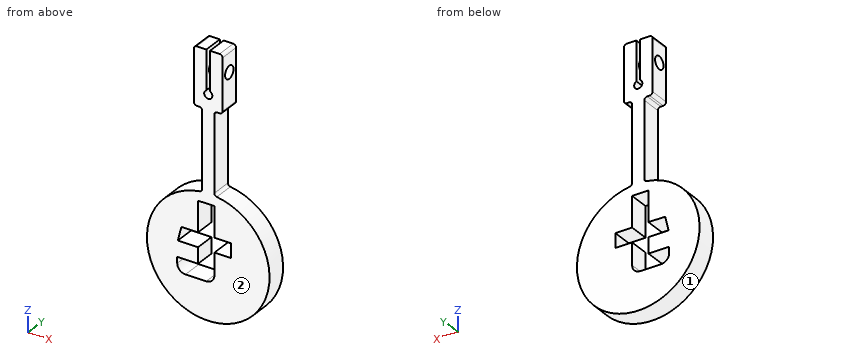
```python
from build123d import *

# Parameters (mm, degrees)
BOSS_EXTRUDE2_DEPTH = 5
SKETCH5_R           = 1.55
CUT_EXTRUDE1_DEPTH  = 60.905859109
FILLET6_R           = 0.7
FILLET7_R           = 0.7
FILLET8_R           = 0.7
FILLET9_R           = 0.7
FILLET10_R          = 0.7
FILLET11_R          = 0.7
FILLET12_R          = 0.7
FILLET13_R          = 0.7
FILLET14_R          = 2
FILLET15_R          = 2


with BuildPart() as part:
    # Sketch3 → Boss-Extrude2 (new body)
    with BuildSketch(Plane(origin=(0, 0, 0), x_dir=(1, 0, 0), z_dir=(0, 1, 0))):
        with BuildLine():
            Line((0.454624582, 2.591384664), (0.454624582, -7))
            Line((0.454624582, -7), (3.5, -7))
            Line((3.5, -7), (3.5, 7))
            Line((3.5, 7), (1.5, 7))
            Line((1.5, 7), (1.5, 26.833112609))
            ThreePointArc((1.5, 26.833112609), (0, 56.757924165), (-1.5, 26.833112609))
            Line((-1.5, 26.833112609), (-1.5, 7))
            Line((-1.5, 7), (-3.5, 7))
            Line((-3.5, 7), (-3.5, -7))
            Line((-3.5, -7), (-0.454624582, -7))
            Line((-0.454624582, -7), (-0.454624582, 2.591384664))
            ThreePointArc((-0.454624582, 2.591384664), (0, 4.482067823), (0.454624582, 2.591384664))
        make_face()
        Polygon((1.5, 36.708863036), (1.5, 29.251163785), (-2.5, 29.251163785), (-2.5, 36.708863036), (-6.573288639, 36.708863036), (-7.435532145, 40.208863036), (-2.5, 40.208863036), (-2.5, 44.101325286), (-7.582366619, 44.101325286), (-7.582366619, 47.601325286), (1.5, 47.601325286), (1.5, 40.208863036), (5.609756824, 40.208863036), (5.609756824, 36.708863036), align=None, mode=Mode.SUBTRACT)
    extrude(amount=BOSS_EXTRUDE2_DEPTH)

    # Sketch5 → Cut-Extrude1 (cut, through all)
    with BuildSketch(Plane.ZY.offset(3.5)):
        with Locations((1.710892138, 2.5)):
            Circle(SKETCH5_R)
    extrude(amount=-CUT_EXTRUDE1_DEPTH, mode=Mode.SUBTRACT)

    # Fillet6
    fillet6_edges = [part.edges().sort_by_distance(p)[0] for p in [
        (1.5, 2.5, -7),
    ]]
    fillet(fillet6_edges, radius=FILLET6_R)

    # Fillet7
    fillet7_edges = [part.edges().sort_by_distance(p)[0] for p in [
        (3.5, 2.5, -7),
    ]]
    fillet(fillet7_edges, radius=FILLET7_R)

    # Fillet8
    fillet8_edges = [part.edges().sort_by_distance(p)[0] for p in [
        (-1.5, 2.5, -7),
    ]]
    fillet(fillet8_edges, radius=FILLET8_R)

    # Fillet9
    fillet9_edges = [part.edges().sort_by_distance(p)[0] for p in [
        (-3.5, 2.5, -7),
    ]]
    fillet(fillet9_edges, radius=FILLET9_R)

    # Fillet10
    fillet10_edges = [part.edges().sort_by_distance(p)[0] for p in [
        (3.5, 2.5, 7),
    ]]
    fillet(fillet10_edges, radius=FILLET10_R)

    # Fillet11
    fillet11_edges = [part.edges().sort_by_distance(p)[0] for p in [
        (-3.5, 2.5, 7),
    ]]
    fillet(fillet11_edges, radius=FILLET11_R)

    # Fillet12
    fillet12_edges = [part.edges().sort_by_distance(p)[0] for p in [
        (1.5, 2.5, -26.833112609),
    ]]
    fillet(fillet12_edges, radius=FILLET12_R)

    # Fillet13
    fillet13_edges = [part.edges().sort_by_distance(p)[0] for p in [
        (-1.5, 2.5, -26.833112609),
    ]]
    fillet(fillet13_edges, radius=FILLET13_R)

    # Fillet14
    fillet14_edges = [part.edges().sort_by_distance(p)[0] for p in [
        (1.5, 2.5, -47.601325286),
    ]]
    fillet(fillet14_edges, radius=FILLET14_R)

    # Fillet15
    fillet15_edges = [part.edges().sort_by_distance(p)[0] for p in [
        (-7.582366619, 2.5, -47.601325286),
    ]]
    fillet(fillet15_edges, radius=FILLET15_R)


solid = part.part
```
The listing builds one solid part. Answer for the finished solid, in the listing's coordinates (mm). Face numbers are marked on the shaded views. Round coordinates to 2 decimals unless told otherwise and drop trailing zeros. Loops run counter-clockwise (first coordinate to the right, second up) from the corner with the lowest first, then second, coordinate; pieces in that order, holes last.
Q1. Section B-B, the plane x = -5 is taken. Determine the outline of the cut face in (y, z).
Q2. Section C-C, the plane y = 2.5 is taken. Count the separate pieces of the cut face and the enclosed holes in it, then the cut area to 3 significant figures.
Q3. Section D-D, the plane z = -33 is taken. Determine the outline of the cut face in (x, y).
Q4. Section A-A, the plane z = -43.5 is taken. Determine the outline of the cut face in (x, y).
Q5. For a pull along X with two mould halves and no side action, classify the marked faces 1 and 2 as released by +X, released by -X, zero draft, split by the parting line, or undercut.
Q6. Find the intervals of material crossed by line 1 (Z direction, x = 0.75, y = 1.8); line 2 (X direction, y = 3.9, z = 2.5); line 3 (X direction, y = 0.5, z = -25.5), in increasing order.
Q7. Given pin 1 Ø2.5 at (x, y) = (-4, 2) entering from -Z; pin 2 Ø1.6 at (y, z) = (1.5, -45) entering from +X; pin 3 Ø1.5 at (y, z) = (3, -34) entering from +X; pin 4 Ø1.6 at (x, z) = (0, -3.48) entering from -Y, each flat-ended and moving along its own axis, determine where each tip first touches the part or whether it passes through.
Completed:
1. outline: (0, -55.9) - (5, -55.9) - (5, -47.6) - (0, -47.6) - close; (0, -44.1) - (5, -44.1) - (5, -40.21) - (0, -40.21) - close; (0, -36.71) - (5, -36.71) - (5, -27.62) - (0, -27.62) - close
2. separate pieces: 3
2. enclosed holes: 1
2. area: 714 mm2
3. outline: (-12.18, 0) - (-2.5, 0) - (-2.5, 5) - (-12.18, 5) - close; (1.5, 0) - (12.18, 0) - (12.18, 5) - (1.5, 5) - close
4. outline: (-14.9, 0) - (-2.5, 0) - (-2.5, 5) - (-14.9, 5) - close; (1.5, 0) - (14.9, 0) - (14.9, 5) - (1.5, 5) - close
5. face 1: split by the parting line
5. face 2: zero draft
6. line 1: z = -56.74 to -47.16, -29.25 to -4.14, -2.82 to 0.33, 3.09 to 7
6. line 2: x = -3.5 to -0.45, 0.45 to 3.5
6. line 3: x = -1.5 to 1.5
7. pin 1: stops at z = -56.5
7. pin 2: stops at x = 14.8
7. pin 3: stops at x = 13.26
7. pin 4: passes through
